Can you work these out from the model? Positions are in its coordinate system, mm. A direction names the side the tool comes from. Coordinates: 2 decimals unless noted, no trailing zeros. Order: outer loops, then holes, each group sorted by start corner. A loop starts at its lowest first (then second) coordinate and runs counter-clockwise, first axis right, second up. Notation, with made-up numbers: M -8.5,8.25 L 34.5,8.25 A13 cw 34.5,14.25 Z; hole C -31,-25.5 d8. An arc over 180 degrees is marked long. Answer as a JSON object with one key per item and string values.
from build123d import *

# Parameters (mm, degrees)
F1_DEPTH       = 25.4
F2_F1_R        = 2.54
F2_F2_R        = 2.54
F3_SIZE        = 5.08
F4_T           = -3.81
F5_R           = 8.89
F6_DEPTH       = 3.81
F7_D           = 5.5
F7_DEPTH       = 12.7
F7_START       = 12.7
F7_CBORE_D     = 9.75
F7_CBORE_DEPTH = 5
F7_TIP         = 1.6523667023


with BuildPart() as f1:
    # F0 (on Right) → F1 (new body)
    with BuildSketch(Plane.YZ):
        Polygon((-190.5, 60.4147898585), (-243.84, 60.4147898585), (-243.84, 9.6147898585), (-50.8, 9.6147898585), (-50.8, 47.7147898585), (-190.5, 47.7147898585), align=None)
    extrude(amount=F1_DEPTH)

    # F2: fillet of radius 2.54 on 5 edges, made by hand

    # F2_f1
    f2_f1_edges = [f1.edges().sort_by_distance(p)[0] for p in [
        (12.7, -190.5, 47.7147898585),
    ]]
    fillet(f2_f1_edges, radius=F2_F1_R)

    # F2_f2
    f2_f2_edges = [f1.edges().sort_by_distance(p)[0] for p in [
        (25.4, -119.38, 47.7147898585),
        (0, -119.38, 47.7147898585),
        (12.7, -50.8, 47.7147898585),
        (12.7, -190.5, 60.4147898585),
        (0, -189.7560512242, 48.4587386342),
        (25.4, -189.7560512242, 48.4587386342),
    ]]
    fillet(f2_f2_edges, radius=F2_F2_R)

    # F3
    f3_edges = [f1.edges().sort_by_distance(p)[0] for p in [
        (25.4, -147.32, 9.61479),
        (12.7, -243.84, 9.61479),
        (12.7, -50.8, 9.61479),
        (0, -147.32, 9.61479),
    ]]
    chamfer(f3_edges, length=F3_SIZE)

    # F4
    f4_openings = [f1.faces().sort_by_distance(p)[0] for p in [
        (12.7, -243.84, 37.55479),
    ]]
    offset(amount=F4_T, openings=f4_openings)

    # F5 (on face) → F6 (cut, through all)
    with BuildSketch(Plane.XY.offset(60.4147898585)):
        with Locations((12.7, -218.1196852207)):
            Circle(F5_R)
    extrude(amount=-F6_DEPTH, mode=Mode.SUBTRACT)

    # F7
    # its depths count from where the whole tool has entered the part; down to there all is cleared
    with Locations(Plane.XY.offset(60.4147898585).offset(-F7_START)):
        with Locations((11.946093291, -120.65)):
            CounterBoreHole(F7_D / 2, F7_CBORE_D / 2, F7_CBORE_DEPTH, depth=F7_DEPTH)
            with Locations((0, 0, -(F7_DEPTH + F7_TIP / 2))):  # 118° drill point
                Cone(0, F7_D / 2, F7_TIP, mode=Mode.SUBTRACT)

    # F8: F1 across face


with BuildPart() as f1_1:
    add(f1.part)
    add(f1.part.mirror(Plane(origin=(12.7, -243.84, 36.5538832465), x_dir=(1, 0, 0), z_dir=(0, -1, 0))))


solid = f1_1.part
Item 1: Which directions (+Z, -Z, +X, -X, +Y, -Y) give clear straight access to the entire face, cutting with the end or side of a thin tool? Please do faces 3 (the cylindrical face through (10.89, -125.41, 45.84)), 4 (the flat face through (13, -190.5, 54)), 5 (the flat face through (13, -293.37, 53)), 6 (the flat face through (13, -245, 60.415)), 7 (the flat face through (17, -368, 47.715)).
Answers follow:
{"face 3": "+Z", "face 4": "+Z, +X, -X, +Y", "face 5": "none", "face 6": "+Z, +X, -X, +Y, -Y", "face 7": "+Z, +X, -X, -Y"}
Item 2: I'm going to push flat-ended pins straight in: pin 1 (3 mm diameter, centred on x = 14.5, z = 55, fed in from -Y); pin 2 (10.5 mm diameter, centred on x = 12.7, y = -269.56, fed in from +Z); pin 3 (2.5 mm diameter, centred on x = 11, z = 52.5, fed in from +Y). Where does each tip first touch, or does it pass through?
Answers follow:
{"pin 1": "stops at y = -297.18", "pin 2": "stops at z = 13.42", "pin 3": "stops at y = -190.5"}
Item 3: Please list where these lines run through material, in increasing order: line 1 (Y direction, x = 12.7, z = 58.4); line 2 (Y direction, x = 20.75, z = 20.5); line 3 (X direction, y = -324, z = 41).
Answers follow:
{"line 1": "y = -297.13 to -278.45, -260.67 to -227.01, -209.23 to -190.55", "line 2": "y = -436.88 to -433.07, -54.61 to -50.8", "line 3": "x = 0 to 3.81, 21.59 to 25.4"}
Item 4: I want a section at A-A, the plane z = 34.5. Write out the boundary of the cut face in (x, y).
Answers follow:
{"outline": "M 0,-436.88 L 25.4,-436.88 L 25.4,-50.8 L 0,-50.8 Z; hole M 3.81,-433.07 L 21.59,-433.07 L 21.59,-54.61 L 3.81,-54.61 Z"}
Item 5: I want a section at D-D, the plane x = 12.25. Give the number of separate pieces and of enclosed holes in the cut face, plus the area to 3 significant figures.
Answers follow:
{"separate pieces": "4", "enclosed holes": "0", "area": "3,040 mm^2"}
Item 6: I want a section at B-B, the plane y = -199.5. Write out the boundary of the cut face in (x, z).
Answers follow:
{"outline": "M 0,14.69 L 5.08,9.61 L 20.32,9.61 L 25.4,14.69 L 25.4,60.41 L 0,60.41 Z; hole M 3.81,16.27 L 6.66,13.42 L 18.74,13.42 L 21.59,16.27 L 21.59,56.6 L 3.81,56.6 Z"}
Item 7: I want a section at C-C, the plane y = -367.03. Write out the boundary of the cut face in (x, z), plus the area to 3 significant figures.
Answers follow:
{"outline": "M 0,14.69 L 5.08,9.61 L 20.32,9.61 L 25.4,14.69 L 25.4,45.17 A2.54 ccw 22.86,47.71 L 16.82,47.71 L 16.82,43.9 L 21.59,43.9 L 21.59,16.27 L 18.74,13.42 L 6.66,13.42 L 3.81,16.27 L 3.81,43.9 L 7.07,43.9 L 7.07,47.71 L 2.54,47.71 A2.54 ccw 0,45.17 Z", "area": "368 mm^2"}
Item 8: If we mould it in two halves opening along X, with no side actions, what happens to faces 1 (the flat face through (12.576, -247.122, 16.8)), 2 (the flat face through (13, -149, 9.615))? For each: pulls with the +X half, pulls with the -X half, needs draft (parallel to the pull), parting line crosses it, or undercut.
Answers follow:
{"face 1": "undercut", "face 2": "needs draft"}
